Input: part model. Units: mm. Frame: model coordinates. A direction names the side the tool comes from. Give positions to 0.01 mm unless a question says otherwise; leave off trailing zeros. Write each loop counter-clockwise with the first axis right and the second up, starting at its lowest first coordinate (ties: lowest second). Pieces come first, ordered by that corner, then holes. Notation, with made-up numbers: (-12, 47) - (3, 47) arc R32 ccw to (3, 76) - close; hole circle Ø1 at (71, 28.25). An arc over 180 degrees is marked (long way). Answer as a JSON object with one key per item and string values. Group by question number.
from build123d import *

# Parameters (mm, degrees)
F1_DEPTH = 37.084


with BuildPart() as f1:
    # F0 (on Front) → F1 (new body)
    with BuildSketch(Plane.XZ):
        with BuildLine():
            ThreePointArc((12.942736, 6.234619), (0.035532, 5.21526), (-10.607814, 12.58779))
            Line((-10.607814, 12.58779), (-10.607814, -6.373834))
            Line((-10.607814, -6.373834), (-7.256928, -6.373834))
            Line((-7.256928, -6.373834), (-7.256928, -3.021034))
            Line((-7.256928, -3.021034), (-5.504328, -3.021034))
            Line((-5.504328, -3.021034), (-5.504328, -6.373834))
            Line((-5.504328, -6.373834), (48.761478, -6.373834))
            Line((48.761478, -6.373834), (48.761478, -3.021034))
            Line((48.761478, -3.021034), (50.546074, -3.021034))
            Line((50.546074, -3.021034), (50.546074, -6.373834))
            Line((50.546074, -6.373834), (60.481984, -6.373834))
            Line((60.481984, -6.373834), (63.549221, -6.373834))
            ThreePointArc((63.549221, -6.373834), (60.255035, -2.563114), (55.918712, 0))
            ThreePointArc((55.918712, 0), (43.08963, 5.393993), (29.482889, 8.31583))
            ThreePointArc((29.482889, 8.31583), (20.855773, 10.112752), (12.942736, 6.234619))
        make_face()
    extrude(amount=F1_DEPTH)


solid = f1.part
1) Mould query, pull axis X, two halves, no side actions, for faces 1 (the face through (-10.608, -18, 3)), 2 (the face through (-9, -18, -6.374)), 3 (the face through (20.981, -18.282, 10.128)). Classes: +X half, -X half, draft (parallel to the pull), parting line (faces both ways), or undercut.
2) Reachability of faces 4 (the face through (-7.257, -18, -5)), 5 (the face through (21, -18, -6.374)) from +Z, -Z, +X, -X, +Y, -Y: full face, straight path, thin tool, end or side. Return the list, or none.
3) Cut plane A-A on y = -28. Return the cut outline in (x, z).
4) Cut plane B-B on z = -4.75. Return the cut outline in (x, y), and give its area (3 significant figures).
5) Cut plane C-C on z = 7. Return the cut outline in (x, y).
6) Line query: line 1 along X through (y, z) = (-16, 8.75); line 2 along X through (y, z) = (-25, -5.5); line 3 along X through (y, z) = (-17, 9). Output: solid intervals per line, ascending. Write a range as from..to.
7) Pin query (flat end, axial travel): P1, Ø1, axis at y = -17.5, z = -4.5, coming from the +X side; P2, Ø1, axis at y = -14.5, z = -5, coming from the +X side; P3, Ø2, axis at x = 28.5, y = -23.5, coming from the +Z side. Return the tip coordinate at first contact, or that it passes through.
8) Cut plane D-D on x = 57. Return the cut outline in (y, z), and give its area (3 significant figures).
Filled in:
{
 "1": {"face 1": "-X half", "face 2": "draft", "face 3": "undercut"},
 "2": {"face 4": "-Z, +Y, -Y", "face 5": "-Z, +X, -X, +Y, -Y"},
 "3": {"outline": "(-10.61, -6.37) - (-7.26, -6.37) - (-7.26, -3.02) - (-5.5, -3.02) - (-5.5, -6.37) - (48.76, -6.37) - (48.76, -3.02) - (50.55, -3.02) - (50.55, -6.37) - (63.55, -6.37) arc R15.61 ccw to (55.92, 0) arc R74.73 ccw to (29.48, 8.32) arc R13.58 ccw to (12.94, 6.23) arc R19.29 cw to (-10.61, 12.59) - close"},
 "4": {"outline": "(-10.61, -37.08) - (-7.26, -37.08) - (-7.26, 0) - (-10.61, 0) - close; (-5.5, -37.08) - (48.76, -37.08) - (48.76, 0) - (-5.5, 0) - close; (50.55, -37.08) - (62.4, -37.08) - (62.4, 0) - (50.55, 0) - close", "area": "2,580 mm²"},
 "5": {"outline": "(-10.61, -37.08) - (-4.35, -37.08) - (-4.35, 0) - (-10.61, 0) - close; (13.77, -37.08) - (37.14, -37.08) - (37.14, 0) - (13.77, 0) - close"},
 "6": {"line 1": "x = -10.61..-6.96, 16.41..28.69", "line 2": "x = -10.61..-7.26, -5.5..48.76, 50.55..62.97", "line 3": "x = -10.61..-7.26, 16.93..28.17"},
 "7": {"P1": "stops at x = 62.6", "P2": "stops at x = 62.97", "P3": "stops at z = 9.28"},
 "8": {"outline": "(-37.08, -6.37) - (0, -6.37) - (0, -0.47) - (-37.08, -0.47) - close", "area": "219 mm²"}
}
